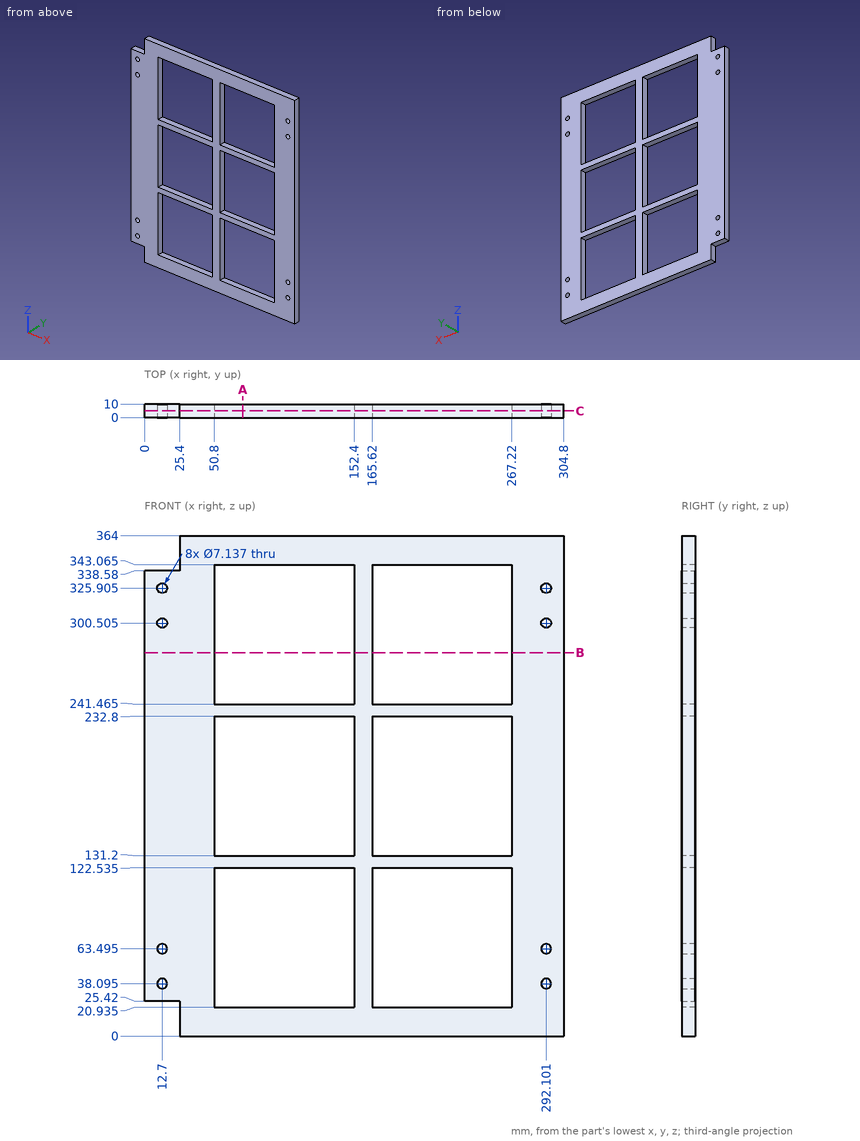
The figure shows three views and two pictorial views of one solid part (mm, origin at its lowest corner). Answer the questions. Round coordinates to 2 decimals unless told otherwise and drop trailing zeros. Write each loop counter-clockwise with the first axis right and the second up, starting at its lowest first coordinate (ties: lowest second). Pieces come first, ordered by that corner, then holes. Notation, with made-up numbers: (72, 77.25) -> (108, 77.25) arc R17 ccw to (108, 90.25) -> close; hole circle Ø5 at (32, 88). An arc over 180 degrees is marked (long way). Answer as a JSON object with one key per item and string values. Group by question number.
Q1. Section B-B (z = 279) is taken. Write down the section's boundary in (x, y).
Q2. Section A-A (x = 71.5) is taken. Write down the section's boundary in (y, z) (1 decimal), plus the area to 3 significant figures.
Q3. Straight lines are drawn through the part: line 1 along X through (y, z) = (4, 249.5); line 2 along Z through (x, y) = (251, 9.75) (1 decimal); line 3 along Z through (x, y) = (289.5, 8). For each, find the intervals that lie inside material, in ascending order.
Q4. Section C-C (y = 5) is taken. Count the separate pieces of the cut face and the enclosed holes in it, plus the area to 3 significant figures.
Check values:
{
 "1": {"outline": "(0, 0) -> (50.8, 0) -> (50.8, 10) -> (0, 10) -> close; (152.4, 0) -> (165.62, 0) -> (165.62, 10) -> (152.4, 10) -> close; (267.22, 0) -> (304.8, 0) -> (304.8, 10) -> (267.22, 10) -> close"},
 "2": {"outline": "(0, 0) -> (10, 0) -> (10, 20.9) -> (0, 20.9) -> close; (0, 122.5) -> (10, 122.5) -> (10, 131.2) -> (0, 131.2) -> close; (0, 232.8) -> (10, 232.8) -> (10, 241.5) -> (0, 241.5) -> close; (0, 343.1) -> (10, 343.1) -> (10, 364) -> (0, 364) -> close", "area": "592 mm^2"},
 "3": {"line 1": "0 to 50.8, 152.4 to 165.62, 267.22 to 304.8", "line 2": "0 to 20.9, 122.5 to 131.2, 232.8 to 241.5, 343.1 to 364", "line 3": "0 to 35.65, 40.54 to 61.05, 65.94 to 298.06, 302.95 to 323.46, 328.35 to 364"},
 "4": {"separate pieces": "1", "enclosed holes": "14", "area": "47,400 mm^2"}
}
